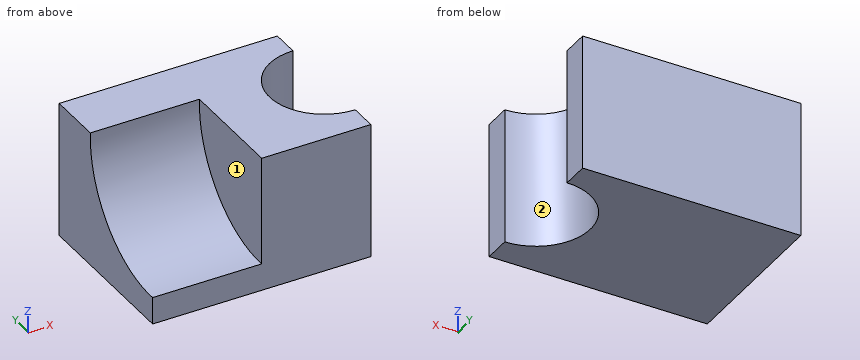
```python
from build123d import *

# Parameters (mm, degrees)
F0_W     = 101.6
F0_H     = 63.5
F1_DEPTH = 76.2
F3_DEPTH = 63.5
F5_DEPTH = 50.8
F7_DEPTH = 50.8


with BuildPart() as f1:
    # F0 (on Front) → F1 (new body)
    with BuildSketch(Plane.XZ):
        with Locations((3.4718271345, -17.4338711586)):
            Rectangle(F0_W, F0_H)
    extrude(amount=F1_DEPTH)

    # F2 (on face) → F3 (cut)
    with BuildSketch(Plane.XY.offset(14.3161288414)):
        with BuildLine():
            Line((54.2718271345, -63.5), (54.2718271345, -12.7))
            ThreePointArc((54.2718271345, -12.7), (28.8718271345, -38.1), (54.2718271345, -63.5))
        make_face()
    extrude(amount=-F3_DEPTH, mode=Mode.SUBTRACT)

    # F4 (on face) → F5 (cut)
    with BuildSketch(Plane(origin=(-47.3281728655, 0, 0), x_dir=(0, -1, 0), z_dir=(-1, 0, 0))):
        with BuildLine():
            ThreePointArc((76.2, -39.4728052417), (114.234520043, -23.7183912016), (129.9889340831, 14.3161288414))
            ThreePointArc((129.9889340831, 14.3161288414), (76.2, 68.1050629246), (22.4110659169, 14.3161288414))
            Line((22.4110659169, 14.3161288414), (76.2, 14.3161288414))
            Line((76.2, 14.3161288414), (76.2, -39.4728052417))
        make_face()
    extrude(amount=-F5_DEPTH, mode=Mode.SUBTRACT)

    # F6 (on face) → F7 (cut)
    with BuildSketch(Plane(origin=(-47.3281728655, 0, 0), x_dir=(0, -1, 0), z_dir=(-1, 0, 0))):
        with BuildLine():
            Line((76.2, 14.3161288414), (25.4, 14.3161288414))
            ThreePointArc((25.4, 14.3161288414), (39.6977680254, -22.1861031331), (76.2, -36.4838711586))
            Line((76.2, -36.4838711586), (76.2, 14.3161288414))
        make_face()
    extrude(amount=-F7_DEPTH, mode=Mode.SUBTRACT)


solid = f1.part
```
Can you work these out from the model? Positions are in its coordinate system, mm. Face numbers are marked on the shaded views. A direction names the side the tool comes from. Coordinates: 2 decimals unless noted, no trailing zeros. Order: outer loops, then holes, each group sorted by start corner. A loop starts at its lowest first (then second) coordinate and runs counter-clockwise, first axis right, second up. Notation, with made-up numbers: (45, 21.5) - (63, 21.5) arc R16 ccw to (63, 31.5) - close; hole circle Ø10 at (-2.75, 85). An arc over 180 degrees is marked (long way). Answer in a Markdown table with one row per item.
1. For pin 1 (3 mm diameter, centred on y = -40.5, z = -25.5, fed in from +X), with a flat end and sliding along its axis, tell me the tip position at first contact or that it passes through.
Reply:
| item | result |
|---|---|
| pin 1 | stops at x = 29.17 |
2. If I drill on line 1 along Y through (x, z) = (-41, 11); line 2 along Y through (x, z) = (44, 0); line 3 along X through (y, z) = (-71, -20), over which ranges is the centre line in solid material (lowest first)?
Reply:
| item | result |
|---|---|
| line 1 | y = -25.38 to 0 |
| line 2 | y = -76.2 to -61.33, -14.87 to 0 |
| line 3 | x = 3.47 to 54.27 |
3. Suppose I cut it at A-A (x = 41). Please give me the cut outline in (y, z), and give its area (3 significant figures).
Reply:
| item | result |
|---|---|
| outline | (-76.2, -49.18) - (-59.76, -49.18) - (-59.76, 14.32) - (-76.2, 14.32) - close; (-16.44, -49.18) - (0, -49.18) - (0, 14.32) - (-16.44, 14.32) - close |
| area | 2,090 mm^2 |
4. Suppose I cut it at D-D (x = -23.5). Please give me the cut outline in (y, z).
Reply:
| item | result |
|---|---|
| outline | (-76.2, -49.18) - (0, -49.18) - (0, 14.32) - (-25.4, 14.32) arc R48.94 cw to (-76.2, -36.48) - close |
5. For the marked faces 1 and 2, which set-ups out of +Z, -Z, +X, -X, +Y, -Y let a thin tool reach every point of the face, with its end or its side?
Reply:
| item | result |
|---|---|
| face 1 | +Z, -X, -Y |
| face 2 | +Z, -Z, +X |
6. Suppose I cut it at C-C (y = -38.1). Please give me the cut outline in (x, z), and give its area (3 significant figures).
Reply:
| item | result |
|---|---|
| outline | (-47.33, -49.18) - (28.87, -49.18) - (28.87, 14.32) - (3.47, 14.32) - (3.47, -20.51) - (-47.33, -20.51) - close |
| area | 3,070 mm^2 |
7. Suppose I cut it at B-B (z = -25.5). Please give me the cut outline in (x, y), and give its area (3 significant figures).
Reply:
| item | result |
|---|---|
| outline | (-47.33, -43.36) - (3.47, -43.36) - (3.47, -76.2) - (54.27, -76.2) - (54.27, -63.5) arc R25.4 cw to (54.27, -12.7) - (54.27, 0) - (-47.33, 0) - close |
| area | 5,060 mm^2 |
